Check sheet for the drawn part. Datum: minimum x, y, z corner. Units: mm. A direction names the side the tool comes from. Round coordinates to 2 decimals unless told otherwise and drop trailing zeros. Write each loop counter-clockwise with the first axis right and the second up, starting at its lowest first coordinate (ties: lowest second). Pieces come first, ordered by that corner, then holes. Notation, with made-up numbers: (50, -35.75) -> (100, -35.75) arc R21 cw to (100, -29.75) -> close; hole circle Ø3 at (28.25, 28). An arc over 180 degrees is marked (long way). One line per item, written item: value. Start each with the question number.
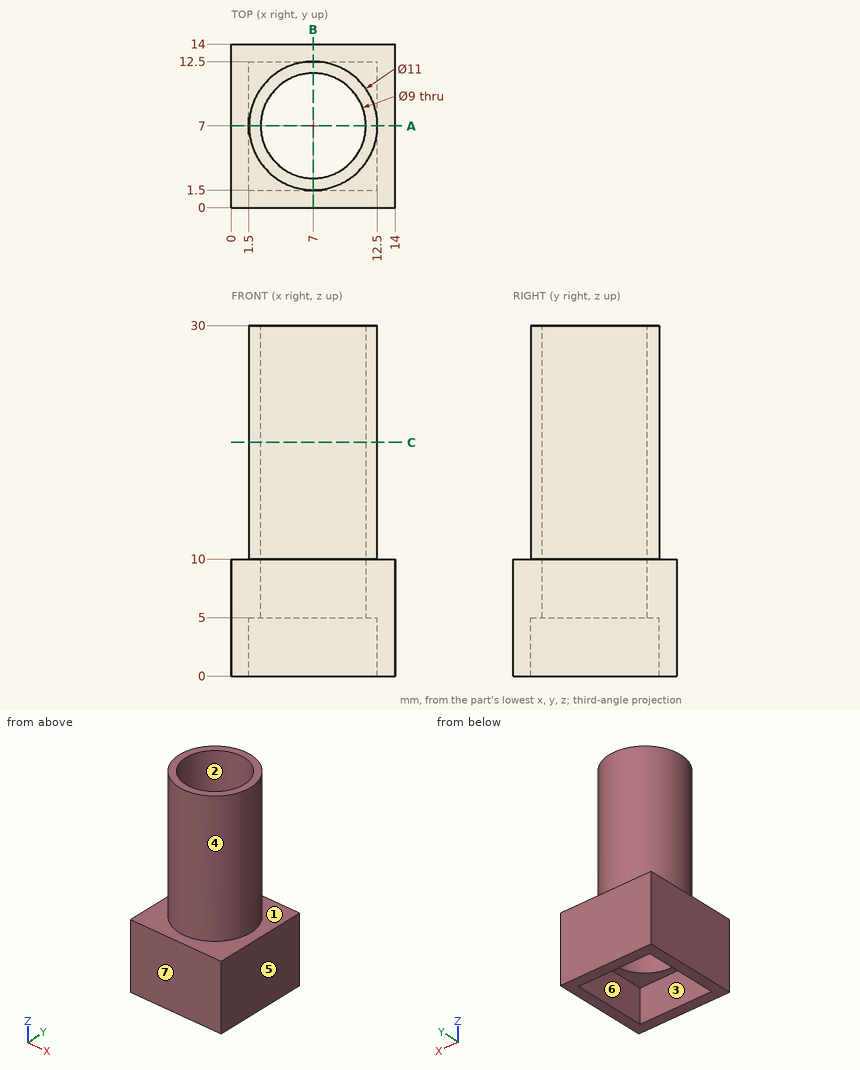
1. Release check for a two-part mould opening along X. For the marked faces 4, 5, 6 and 7 record: +X half, -X half, draft (parallel to the pull), parting line (faces both ways), or undercut.
2. Cross-section at A-A (y = 7). Record the cut outline in (x, z), plus the area to 3 significant figures.
3. Depth check by flat-ended pin: pin 1 Ø8 at (x, z) = (6.5, 20.5) entering from +Y; pin 2 Ø1 at (x, y) = (4.5, 6.5) entering from +Z; pin 3 Ø1 at (x, z) = (3.5, 14) entering from +Y; pin 4 Ø8 at (x, z) = (8.5, 23) entering from -Y. Enter the tip coordinate at first touch or a pass-through.
4. Material ranges on probe 1 along Y at (x, z) = (10.75, 3); probe 2 along Y at (x, z) = (7, 18.5); probe 3 along X at (y, z) = (7.5, 25.5), recorded low to high.
5. Cross-section at C-C (z = 20). Record the cut outline in (x, y), plus the area to 3 significant figures.
6. Access from +Z, -Z, +X, -X, +Y, -Y to the whole of each face (thin tool, end or side, straight path). Record for the marked faces 1, 2 and 3.
Working result:
1. face 4: parting line
1. face 5: +X half
1. face 6: undercut
1. face 7: draft
2. outline: (0, 0) -> (1.5, 0) -> (1.5, 5) -> (2.5, 5) -> (2.5, 30) -> (1.5, 30) -> (1.5, 10) -> (0, 10) -> close; (11.5, 5) -> (12.5, 5) -> (12.5, 0) -> (14, 0) -> (14, 10) -> (12.5, 10) -> (12.5, 30) -> (11.5, 30) -> close
2. area: 80.0 mm^2
3. pin 1: stops at y = 12.5
3. pin 2: passes through
3. pin 3: stops at y = 11.61
3. pin 4: stops at y = 1.5
4. probe 1: y = 0 to 1.5, 12.5 to 14
4. probe 2: y = 1.5 to 2.5, 11.5 to 12.5
4. probe 3: x = 1.52 to 2.53, 11.47 to 12.48
5. outline: circle Ø11 at (7, 7); hole circle Ø9 at (7, 7)
5. area: 31.4 mm^2
6. face 1: +Z
6. face 2: +Z, -Z
6. face 3: -Z
